Drawing for the job (mm, zero at the part's lowest x, y, z). Coordinates: 2 decimals unless noted, no trailing zeros. Loops run counter-clockwise (first coordinate to the right, second up) from the corner with the lowest first, then second, coordinate; pieces in that order, holes last.
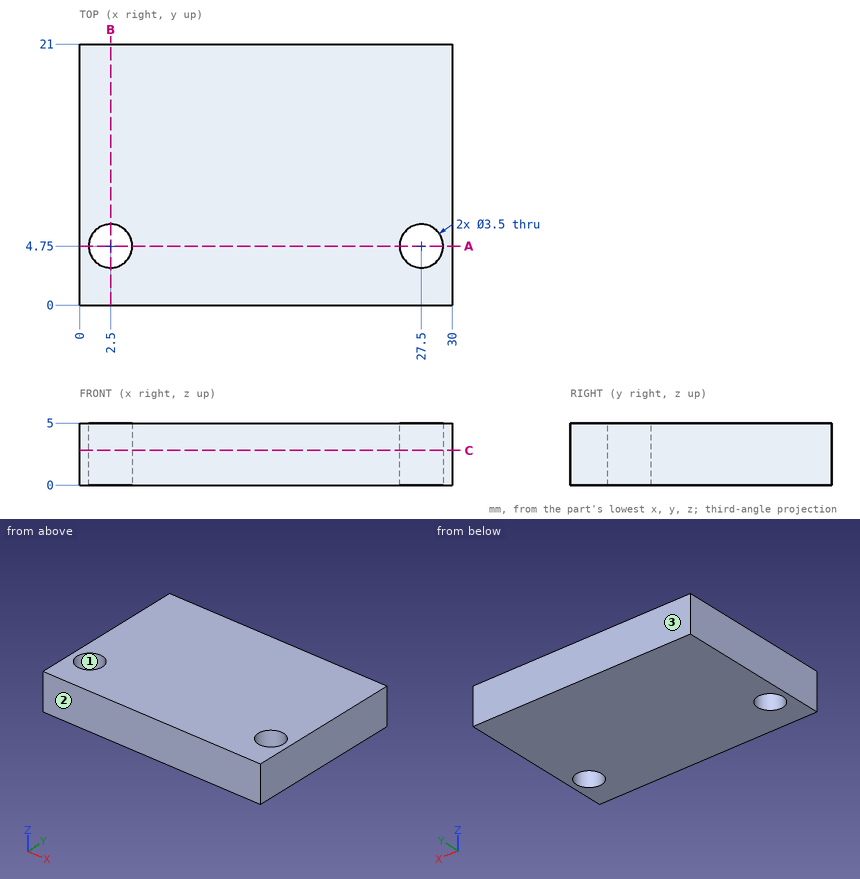
Q1. Saw through at C-C (z = 2.8). List the corners of the cut face in (x, y), plus the area to 3 significant figures.
Q2. Probe line 1 (Y direction, x = 27.5, z = 1.9); line 2 (X direction, y = 3.5, z = 2.2); line 3 (X direction, y = 4, z = 0.3). List the from-to ranges inside material, lowest first.
Q3. Saw through at B-B (x = 2.5). List the corners of the cut face in (y, z), plus the area to 3 significant figures.
Q4. Saw through at A-A (y = 4.75). List the corners of the cut face in (x, z), plus the area to 3 significant figures.
Q5. Mould opens along Y. For the marked faces 1, 2 and 3 say: released by +Y, released by -Y, zero draft, split by the parting line, or undercut.
Checked values:
1. outline: (0, 0) - (30, 0) - (30, 21) - (0, 21) - close; hole circle Ø3.5 at (2.5, 4.75); hole circle Ø3.5 at (27.5, 4.75)
1. area: 611 mm2
2. line 1: y = 0 to 3, 6.5 to 21
2. line 2: x = 0 to 1.28, 3.72 to 26.28, 28.72 to 30
2. line 3: x = 0 to 0.92, 4.08 to 25.92, 29.08 to 30
3. outline: (0, 0) - (3, 0) - (3, 5) - (0, 5) - close; (6.5, 0) - (21, 0) - (21, 5) - (6.5, 5) - close
3. area: 87.5 mm2
4. outline: (0, 0) - (0.75, 0) - (0.75, 5) - (0, 5) - close; (4.25, 0) - (25.75, 0) - (25.75, 5) - (4.25, 5) - close; (29.25, 0) - (30, 0) - (30, 5) - (29.25, 5) - close
4. area: 115 mm2
5. face 1: undercut
5. face 2: released by -Y
5. face 3: released by +Y
